Could you check a few things on this drawing? It's one solid part, dimensions in mm from its lowest x, y, z. A direction names the side the tool comes from. Give positions to 0.01 mm unless a question says otherwise; leave off trailing zeros. Loops run counter-clockwise (first coordinate to the right, second up) from the corner with the lowest first, then second, coordinate; pieces in that order, holes last. Notation, with made-up numbers: (-28.5, -33) - (-11.5, -33) arc R24 cw to (-11.5, -3) - close; hole circle Ø6 at (14, 69.5). An arc over 180 degrees is marked (long way). Put each result on its own line as item: value. Start each with the question number.
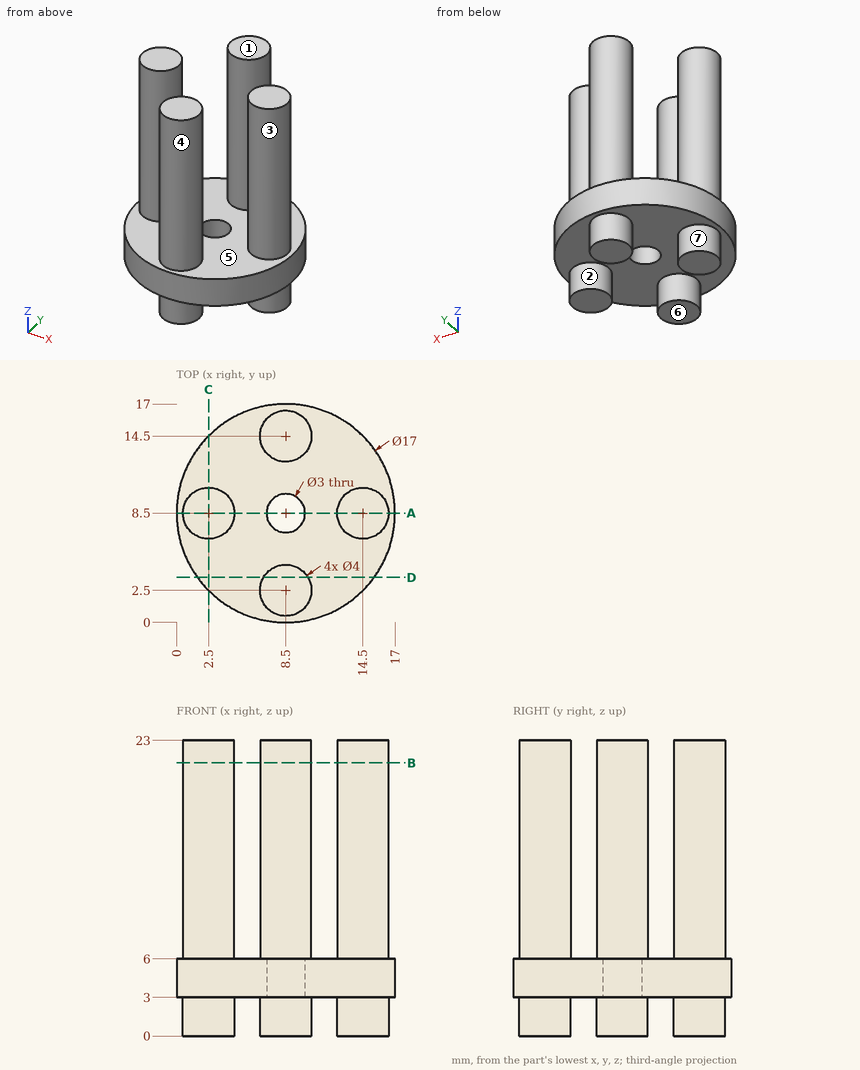
1) Suppose I cut it at B-B on z = 21.25. Please give me the cut outline in (x, y).
2) Suppose I cut it at A-A on y = 8.5. Please give me the cut outline in (x, z), plus the area to 3 significant figures.
3) Which directions (+Z, -Z, +X, -X, +Y, -Y) give clear straight access to the entire face, cutting with the end or side of a thin tool? Please do the marked faces 5, 6 and 7.
4) Suppose I cut it at C-C on x = 2.5. Please give me the cut outline in (y, z), plus the area to 3 significant figures.
5) Suppose I cut it at D-D on y = 3.5. Please give me the cut outline in (x, z), plus the area to 3 significant figures.
6) I need wall thicknesses on line 1 (Y direction, x = 8.5, z = 4.85); line 2 (Z direction, x = 13, y = 6.5); line 3 (X direction, y = 8, z = 13.5). Which ranges of each line are inside material? Lowest first, please.
7) Thinking about a two-plate mould opening in X: for the marked faces 1, 2, 3 and 4, which applies, pulls with the +X half, pulls with the -X half, needs draft (parallel to the pull), parting line crosses it, or undercut?
8) I'm going to push flat-ended pins straight in: P1, Ø1, axis at y = 15, z = 11.5, coming from the -X side; P2, Ø6, axis at x = 7, z = 14.5, coming from the +Y side; P3, Ø6, axis at y = 13, z = 4, coming from the +X side. Where does each tip first touch, or does it pass through?
Ans:
1. outline: circle Ø4 at (2.5, 8.5); circle Ø4 at (8.5, 2.5); circle Ø4 at (8.5, 14.5); circle Ø4 at (14.5, 8.5)
2. outline: (0, 3) - (0.5, 3) - (0.5, 0) - (4.5, 0) - (4.5, 3) - (7, 3) - (7, 6) - (4.5, 6) - (4.5, 23) - (0.5, 23) - (0.5, 6) - (0, 6) - close; (10, 3) - (12.5, 3) - (12.5, 0) - (16.5, 0) - (16.5, 3) - (17, 3) - (17, 6) - (16.5, 6) - (16.5, 23) - (12.5, 23) - (12.5, 6) - (10, 6) - close
2. area: 202 mm²
3. face 5: +Z
3. face 6: -Z, +X, -X, +Y, -Y
3. face 7: -Z
4. outline: (2.48, 3) - (6.5, 3) - (6.5, 0) - (10.5, 0) - (10.5, 3) - (14.52, 3) - (14.52, 6) - (10.5, 6) - (10.5, 23) - (6.5, 23) - (6.5, 6) - (2.48, 6) - close
4. area: 116 mm²
5. outline: (1.63, 3) - (6.77, 3) - (6.77, 0) - (10.23, 0) - (10.23, 3) - (15.37, 3) - (15.37, 6) - (10.23, 6) - (10.23, 23) - (6.77, 23) - (6.77, 6) - (1.63, 6) - close
5. area: 111 mm²
6. line 1: y = 0 to 7, 10 to 17
6. line 2: z = 3 to 6
6. line 3: x = 0.56 to 4.44, 12.56 to 16.44
7. face 1: needs draft
7. face 2: undercut
7. face 3: undercut
7. face 4: parting line crosses it
8. P1: stops at x = 6.5
8. P2: stops at y = 16.5
8. P3: stops at x = 16.87
